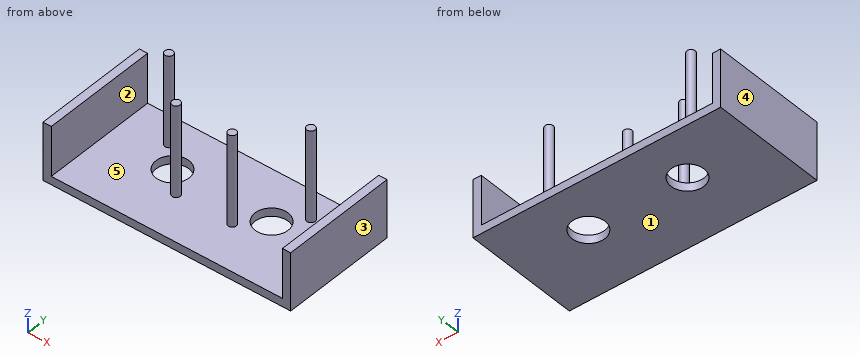
from build123d import *

# Parameters (mm, degrees)
ESQUISSE1_W             = 150
ESQUISSE1_H             = 70
BOSS_EXTRU_1_DEPTH      = 5
ESQUISSE2_W             = 5
ESQUISSE2_H             = 70
BOSS_EXTRU_2_DEPTH      = 30
ESQUISSE3_R             = 10
ENL_V_MAT_EXTRU_1_DEPTH = 30
ESQUISSE5_R             = 2.5
BOSS_EXTRU_3_DEPTH      = 60


with BuildPart() as part:
    # Esquisse1 → Boss.-Extru.1 (new body)
    with BuildSketch(Plane.XY):
        with Locations((8.080821687, -0.482695652)):
            Rectangle(ESQUISSE1_W, ESQUISSE1_H)
    extrude(amount=BOSS_EXTRU_1_DEPTH)

    # Esquisse2 → Boss.-Extru.2 (add)
    with BuildSketch(Plane.XY.offset(5)):
        with Locations((-64.419178313, -0.482695652)):
            Rectangle(ESQUISSE2_W, ESQUISSE2_H)
        with Locations((80.580821687, -0.482695652)):
            Rectangle(ESQUISSE2_W, ESQUISSE2_H)
    extrude(amount=BOSS_EXTRU_2_DEPTH)

    # Esquisse3 → Enlèv. mat.-Extru.1 (cut)
    with BuildSketch(Plane(origin=(0, 0, 0), x_dir=(-1, 0, 0), z_dir=(0, 0, -1))):
        with Locations((21.919178313, 4.647304348)):
            Circle(ESQUISSE3_R)
        with Locations((-38.080821687, 4.647304348)):
            Circle(ESQUISSE3_R)
    extrude(amount=-ENL_V_MAT_EXTRU_1_DEPTH, mode=Mode.SUBTRACT)

    # Esquisse5 → Boss.-Extru.3 (add)
    with BuildSketch(Plane(origin=(0, 0, 0), x_dir=(-1, 0, 0), z_dir=(0, 0, -1))):
        with Locations((34.919178313, 17.647304348)):
            Circle(ESQUISSE5_R)
        with Locations((8.919178313, -8.352695652)):
            Circle(ESQUISSE5_R)
        with Locations((-51.080821687, 17.647304348)):
            Circle(ESQUISSE5_R)
        with Locations((-25.080821687, -8.352695652)):
            Circle(ESQUISSE5_R)
    extrude(amount=-BOSS_EXTRU_3_DEPTH)


solid = part.part
Can you work these out from the model? Positions are in its coordinate system, mm. Face numbers are marked on the shaded views. A direction names the side the tool comes from. Coordinates: 2 decimals unless noted, no trailing zeros. Write each loop counter-clockwise with the first axis right and the second up, starting at its lowest first coordinate (ties: lowest second). Pieces come first, ordered by that corner, then holes. Notation, with made-up numbers: (60.5, -24.75) -> (93.5, -24.75) arc R30 cw to (93.5, 5.25) -> close; hole circle Ø9 at (76.25, 45.5). An arc over 180 degrees is marked (long way). Write each question's results on one line, items separated by ' | '. Start each with the question number.
Item 1: Please list where these lines run through material, in increasing order: probe 1 along X at (y, z) = (24, 14); probe 2 along X at (y, z) = (16.5, 22.5); probe 3 along Z at (x, y) = (49, 5).
Item 2: If we section it at B-B, the plane y = -21: Write out the boundary of the cut face in (x, z).
Item 3: I'm going to push flat-ended pins straight in: P1, Ø4, axis at x = -1.5, y = 13, coming from the -Z side; P2, Ø23, axis at x = 38.08, y = 4.65, coming from the +Z side; P3, Ø6, axis at x = 49.5, z = 17.5, coming from the -Y side; P4, Ø4, axis at x = 80.5, y = -12, coming from the +Z side. Where does each tip first touch, or does it pass through?
Item 4: On a 3-axis mill with a long thin cutter (end or side, diameter ignored), from which of +Z, -Z, +X, -X, +Y, -Y can I reach the whole of each face in a straight line? I mean the marked faces 1 and 2. Say none if no direction works.
Item 5: If we section it at C-C, the plane z = 21.5: Write out the boundary of the cut face in (x, y).
Item 6: Thinking about a two-plate mould opening in X: for the marked faces 3, 4 and 5, which applies, released by +X, released by -X, zero draft, split by the parting line, or undercut?
Item 7: If we section it at A-A, the plane x = 41.5: Write out the boundary of the cut face in (y, z), and give its area (3 significant figures).
Item 8: If we section it at D-D, the plane y = -2.5: Write out the boundary of the cut face in (x, z).
Answer block:
1) probe 1: -66.92 to -61.92, 78.08 to 83.08 | probe 2: -66.92 to -61.92, -37.14 to -32.7, 48.86 to 53.3, 78.08 to 83.08 | probe 3: 0 to 5
2) outline: (-66.92, 0) -> (83.08, 0) -> (83.08, 35) -> (78.08, 35) -> (78.08, 5) -> (-61.92, 5) -> (-61.92, 35) -> (-66.92, 35) -> close
3) P1: z = 0 | P2: z = 5 | P3: y = 15.15 | P4: z = 35
4) face 1: -Z, +X, -X, +Y, -Y | face 2: +Z, +Y, -Y
5) outline: (-66.92, -35.48) -> (-61.92, -35.48) -> (-61.92, 34.52) -> (-66.92, 34.52) -> close; circle Ø5 at (-34.92, 17.65); circle Ø5 at (-8.92, -8.35); circle Ø5 at (25.08, -8.35); circle Ø5 at (51.08, 17.65); (78.08, -35.48) -> (83.08, -35.48) -> (83.08, 34.52) -> (78.08, 34.52) -> close
6) face 3: released by +X | face 4: released by -X | face 5: undercut
7) outline: (-35.48, 0) -> (-4.75, 0) -> (-4.75, 5) -> (-35.48, 5) -> close; (14.04, 0) -> (34.52, 0) -> (34.52, 5) -> (14.04, 5) -> close | area: 256 mm²
8) outline: (-66.92, 0) -> (-28.91, 0) -> (-28.91, 5) -> (-61.92, 5) -> (-61.92, 35) -> (-66.92, 35) -> close; (-14.93, 0) -> (31.09, 0) -> (31.09, 5) -> (-14.93, 5) -> close; (45.07, 0) -> (83.08, 0) -> (83.08, 35) -> (78.08, 35) -> (78.08, 5) -> (45.07, 5) -> close
